Part model, mm, in its own coordinate system. Round coordinates to 2 decimals unless told otherwise and drop trailing zeros. Loops run counter-clockwise (first coordinate to the right, second up) from the corner with the lowest first, then second, coordinate; pieces in that order, holes last.
Autodesk Inventor part; units mm, degrees
ref_plane "YZ Plane" through (0, 0, 0) normal (1, 0, 0) x (0, 1, 0)
ref_plane "XZ Plane" through (0, 0, 0) normal (0, 1, 0) x (-1, 0, 0)
ref_plane "XY Plane" through (0, 0, 0) normal (0, 0, 1) x (1, 0, 0)
sketch "Sketch1" plane through (0, 0, 0) normal (0, 0, 1) x (1, 0, 0)
  line L0 (-58.4821, 15.1494) -> (125.7179, 15.1494)
  line L1 (125.7179, 15.1494) -> (125.7179, -11.7506)
  line L2 (125.7179, -11.7506) -> (-58.4821, -11.7506)
  line L3 (-58.4821, -11.7506) -> (-58.4821, 15.1494)
  point P0 (0, 0)
  dimension "d0" = 184.2
  dimension "d2" = 26.9
extrude "Extrusion1" add sketch "Sketch1" along normal blind 1.9
sketch "Sketch5" plane through (0, 0, 1.9) normal (0, 0, 1) x (1, 0, 0)
  line L0 (-58.4821, 15.1494) -> (-58.4821, -11.7506)
  line L1 (-58.4821, -11.7506) -> (125.7179, -11.7506)
  line L2 (125.7179, -11.7506) -> (125.7179, 15.1494)
  circle A0 centre (-25.9821, -2.0006) radius 3.5
  circle A1 centre (-14.7321, -2.0006) radius 2.5
  circle A2 centre (-6.9321, -2.5006) radius 1.9
  circle A3 centre (-6.9321, 2.6994) radius 1.9
  line L3 (8.5679, -2.7506) -> (35.1679, -2.7506)
  line L4 (35.1679, -2.7506) -> (35.1679, 7.1494)
  line L5 (35.1679, 7.1494) -> (8.5679, 7.1494)
  line L6 (8.5679, 7.1494) -> (8.5679, -2.7506)
  line L7 (59.0179, -2.7506) -> (85.6179, -2.7506)
  line L8 (85.6179, -2.7506) -> (85.6179, 7.1494)
  line L9 (85.6179, 7.1494) -> (59.0179, 7.1494)
  line L10 (59.0179, 7.1494) -> (59.0179, -2.7506)
  point P0 (0, 0)
  dimension "d56" = 7
  dimension "d58" = 5
  dimension "d59" = 32.5
  dimension "d60" = 43.75
  dimension "d61" = 9.75
  dimension "d62" = 9.75
  dimension "d63" = 3.8
  dimension "d64" = 3.8
  dimension "d65" = 51.55
  dimension "d66" = 51.55
  dimension "d67" = 9.25
  dimension "d68" = 14.45
  dimension "d69" = 26.6
  dimension "d70" = 26.6
  dimension "d71" = 9.9
  dimension "d72" = 9.9
  dimension "d73" = 9
  dimension "d74" = 9
  dimension "d75" = 117.15
  dimension "d76" = 66.7
extrude "Extrusion3" cut sketch "Sketch5" against normal through all
equation "\"BendRadius\" = Thickness"
equation "\"BendReliefWidth\" = Thickness"
equation "\"BendReliefDepth\" = 0.5 * Thickness"
equation "\"CornerReliefSize\" = 4 * Thickness"
equation "\"MinimumRemnant\" = 2 * Thickness"
equation "\"TransitionRadius\" = BendRadius"
equation "\"JacobiRadiusSize\" = BendRadius"
equation "\"GapSize\" = Thickness"
properties part number "panel"
1) Drop flat-ended pins along their axis: pin 1 Ø6.5 at (x, y) = (-25.98, -2) entering from -Z; pin 2 Ø12 at (x, y) = (18, 7) entering from -Z. Give the stop position or say it passes through.
Values:
pin 1: passes through
pin 2: stops at z = 0
2) Slice it at B-B, the plane z = 1.25. Give the cut face in (x, y).
Values:
outline: (-58.48, -11.75) - (125.72, -11.75) - (125.72, 15.15) - (-58.48, 15.15) - close; hole circle Ø7 at (-25.98, -2); hole circle Ø5 at (-14.73, -2); hole circle Ø3.8 at (-6.93, -2.5); hole circle Ø3.8 at (-6.93, 2.7); hole (8.57, -2.75) - (35.17, -2.75) - (35.17, 7.15) - (8.57, 7.15) - close; hole (59.02, -2.75) - (85.62, -2.75) - (85.62, 7.15) - (59.02, 7.15) - close
3) Slice it at A-A, the plane x = 74. Give the cut face in (y, z).
Values:
outline: (-11.75, 0) - (-2.75, 0) - (-2.75, 1.9) - (-11.75, 1.9) - close; (7.15, 0) - (15.15, 0) - (15.15, 1.9) - (7.15, 1.9) - close
4) Wall check: line 1 along X through (y, z) = (-2.25, 1.7); line 2 along X through (y, z) = (6, 0.3); line 3 along Y through (x, z) = (-23.5, 0.75). Give the ranges that are in metal, low to high.
Values:
line 1: x = -58.48 to -29.47, -22.49 to -17.22, -12.24 to -8.82, -5.05 to 8.57, 35.17 to 59.02, 85.62 to 125.72
line 2: x = -58.48 to 8.57, 35.17 to 59.02, 85.62 to 125.72
line 3: y = -11.75 to -4.47, 0.47 to 15.15
5) Mould opens along X. For faces 1 (the face through (32, 8, 1.9)), 2 (the face through (-5.12, -1.93, 0.96)), 3 (the face through (-12.348, -1.25, 0.963)) say: released by +X, released by -X, zero draft, split by the parting line, or undercut.
Values:
face 1: zero draft
face 2: undercut
face 3: undercut
